CAD build for the part. Positions are in the model's coordinates, mm. Round coordinates to 2 decimals unless told otherwise and drop trailing zeros. Write each loop counter-clockwise with the first axis right and the second up, starting at its lowest first coordinate (ties: lowest second). Pieces come first, ordered by that corner, then holes. Notation, with made-up numbers: (85.25, -16) - (104.25, -16) arc R17 ccw to (104.25, 16) - close; hole circle Ø6 at (38, 13). An arc over 180 degrees is marked (long way). Use one line per item in the form item = value. Start each with the question number.
Item 1: Band-saw the part on A-A, the plane x = 65. List the corners of the cut face in (y, z), and give its area (3 significant figures).
Item 2: Pull direction X, two halves, no side cores. Call faces 1 (the flat face through (35, 0, -106)), 2 (the cylindrical face through (63, 1, -5)): +X half, -X half, draft (parallel to the pull), parting line (faces both ways), or undercut.
Item 3: Pin check, flat tip, straight feed: pin 1 (2 mm diameter, centred on x = 17.5, z = -5, fed in from -Y). Stop position of the tip, or through.
Item 4: Drill centre lines: L1, parallel to Z at x = 65, y = 1.1; L2, parallel to X at y = 0.6, z = -5; L3, parallel to Z at x = 17.5, y = 1.25. Where is each one in solid material? Low to high.
from build123d import *

# Parameters (mm, degrees)
SKETCH1_W               = 70
SKETCH1_H               = 210
BOSS_EXTRUDE1_DEPTH     = 2
SKETCH2_R               = 2
CUT_EXTRUDE1_DEPTH      = 3
TAP_DRILL_FOR_M3_TAP1_D = 2.5
TAP_DRILL_FOR_M3_TAP2_D = 2.5
TAP_DRILL_FOR_M3_TAP3_D = 2.5


with BuildPart() as part:
    # Sketch1 → Boss-Extrude1 (new body)
    with BuildSketch(Plane(origin=(0, 0, 0), x_dir=(1, 0, 0), z_dir=(0, 1, 0))):
        with Locations((35, 105)):
            Rectangle(SKETCH1_W, SKETCH1_H)
    extrude(amount=BOSS_EXTRUDE1_DEPTH)

    # Sketch2 → Cut-Extrude1 (cut, through all)
    with BuildSketch(Plane(origin=(0, 2, 0), x_dir=(1, 0, 0), z_dir=(0, 1, 0))):
        with Locations((5, 205)):
            Circle(SKETCH2_R)
        with Locations((65, 205)):
            Circle(SKETCH2_R)
        with Locations((65, 5)):
            Circle(SKETCH2_R)
        with Locations((5, 5)):
            Circle(SKETCH2_R)
    extrude(amount=-CUT_EXTRUDE1_DEPTH, mode=Mode.SUBTRACT)

    # Tap Drill for M3 Tap1 (through all)
    with Locations(Plane(origin=(0, 2, 0), x_dir=(1, 0, 0), z_dir=(0, 1, 0))):
        with Locations((35, 205), (35, 130.3), (35, 55.6)):
            Hole(TAP_DRILL_FOR_M3_TAP1_D / 2)

    # Tap Drill for M3 Tap2 (through all)
    with Locations(Plane(origin=(0, 2, 0), x_dir=(1, 0, 0), z_dir=(0, 1, 0))):
        with Locations((52.5, 5), (17.5, 5), (17.5, 40), (52.5, 40)):
            Hole(TAP_DRILL_FOR_M3_TAP2_D / 2)

    # Tap Drill for M3 Tap3 (through all)
    with Locations(Plane(origin=(0, 2, 0), x_dir=(1, 0, 0), z_dir=(0, 1, 0))):
        with Locations((19.9, 26.6), (50.1, 11)):
            Hole(TAP_DRILL_FOR_M3_TAP3_D / 2)


solid = part.part
Determined:
q1.outline = (0, -210) - (2, -210) - (2, -207) - (0, -207) - close; (0, -203) - (2, -203) - (2, -7) - (0, -7) - close; (0, -3) - (2, -3) - (2, 0) - (0, 0) - close
q1.area = 404 mm²
q2.face_1 = draft
q2.face_2 = undercut
q3.pin_1 = through
q4.L1 = -210 to -207, -203 to -7, -3 to 0
q4.L2 = 0 to 3, 7 to 16.25, 18.75 to 51.25, 53.75 to 63, 67 to 70
q4.L3 = -210 to -41.25, -38.75 to -6.25, -3.75 to 0
